Verification items for the finished model (mm, model axes). Face numbers are marked on the shaded views. A direction names the side the tool comes from. Coordinates: 2 decimals unless noted, no trailing zeros. Write each loop counter-clockwise with the first axis right and the second up, starting at its lowest first coordinate (ties: lowest second). Pieces come first, ordered by that corner, then holes. Notation, with made-up numbers: (83.25, 15) -> (114.25, 15) arc R22 cw to (114.25, 31) -> close; hole circle Ø8 at (38.25, -0.75). An arc over 180 degrees is marked (long way). Answer in a Markdown table with one row per item.
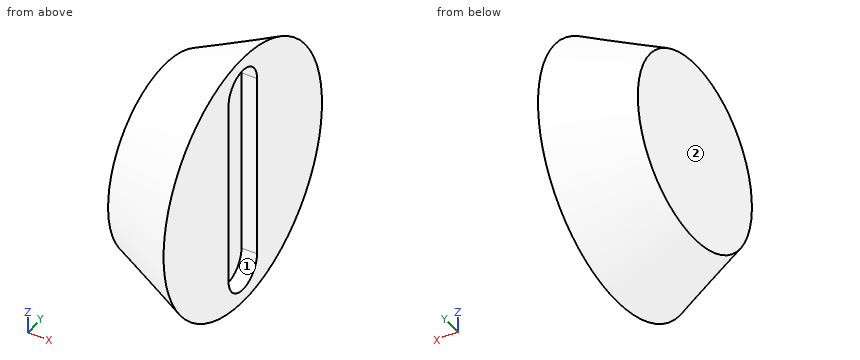
```python
from build123d import *

# Parameters (mm, degrees)
SKETCH1_R           = 30
BOSS_EXTRUDE1_DEPTH = 25
BOSS_EXTRUDE1_DRAFT = -25
CUT_EXTRUDE1_DEPTH  = 5


with BuildPart() as part:
    # Sketch1 → Boss-Extrude1 (with draft: the straight prism first)
    with BuildSketch(Plane(origin=(0, 0, 0), x_dir=(0, 0, -1), z_dir=(1, 0, 0))):
        Circle(SKETCH1_R)
    extrude(amount=BOSS_EXTRUDE1_DEPTH)
    # Boss-Extrude1: the draft: its side faces are tilted about the plane it starts from
    boss_extrude1_sides = [part.faces().sort_by_distance(p)[0] for p in [
        (12.5, 0, 30),
    ]]
    draft(boss_extrude1_sides, Plane(origin=(0, 0, 0), x_dir=(0, 0, -1), z_dir=(1, 0, 0)), BOSS_EXTRUDE1_DRAFT)

    # Sketch2 → Cut-Extrude1 (cut)
    with BuildSketch(Plane(origin=(25, 0, 0), x_dir=(0, 0, -1), z_dir=(1, 0, 0))):
        with BuildLine():
            Line((-30, 7.5), (30, 7.5))
            ThreePointArc((30, 7.5), (37.5, 0), (30, -7.5))
            Line((30, -7.5), (-30, -7.5))
            ThreePointArc((-30, -7.5), (-37.5, 0), (-30, 7.5))
        make_face()
    extrude(amount=-CUT_EXTRUDE1_DEPTH, mode=Mode.SUBTRACT)


solid = part.part
```
1. Material ranges on probe 1 along Y at (x, z) = (22.25, -26); probe 2 along Y at (x, z) = (21, 1); probe 3 along X at (y, z) = (-4, -24), recorded low to high. Write a range as from..to.
Findings below:
| item | result |
|---|---|
| probe 1 | y = -30.89..-7.5, 7.5..30.89 |
| probe 2 | y = -39.78..-7.5, 7.5..39.78 |
| probe 3 | x = 0..20 |
2. Sectioned sample at D-D, the plane x = 4.5. Record the cut outline in (y, z), and give its area (3 significant figures).
Findings below:
| item | result |
|---|---|
| outline | circle Ø64.2 at (0, 0) |
| area | 3,240 mm² |
3. Sectioned sample at C-C, the plane x = 21.25. Record the cut outline in (y, z), and give its area (3 significant figures).
Findings below:
| item | result |
|---|---|
| outline | circle Ø79.82 at (0, 0); hole (-7.5, -30) arc R7.5 ccw to (7.5, -30) -> (7.5, 30) arc R7.5 ccw to (-7.5, 30) -> close |
| area | 3,930 mm² |
4. Sectioned sample at B-B, the plane z = 0. Record the cut outline in (x, y).
Findings below:
| item | result |
|---|---|
| outline | (0, -30) -> (25, -41.66) -> (25, -7.5) -> (20, -7.5) -> (20, 7.5) -> (25, 7.5) -> (25, 41.66) -> (0, 30) -> close |
5. Go/stop test with flat-tipped pins: pin 1 (8 mm diameter, centred on y = 0.5, z = 10, fed in from +X); pin 2 (6 mm diameter, centred on x = 17, z = 14, fed in from -Y); pin 3 (4 mm diameter, centred on x = 13.5, y = 25.5, fed in from +Z) (3 decimals). Record where each tip stops, or that it passes through.
Findings below:
| item | result |
|---|---|
| pin 1 | stops at x = 20 |
| pin 2 | stops at y = -37.09 |
| pin 3 | stops at z = 28.055 |
6. Access from +Z, -Z, +X, -X, +Y, -Y to the whole of each face (thin tool, end or side, straight path). Record for the marked faces 1 and 2.
Findings below:
| item | result |
|---|---|
| face 1 | +X |
| face 2 | +Z, -Z, -X, +Y, -Y |
7. Sectioned sample at A-A, the plane y = 0. Record the cut outline in (x, z).
Findings below:
| item | result |
|---|---|
| outline | (0, -30) -> (25, -41.66) -> (25, -37.5) -> (20, -37.5) -> (20, 37.5) -> (25, 37.5) -> (25, 41.66) -> (0, 30) -> close |
